Build history of the part. All positions in model axes, mm. A direction names the side the tool comes from. Give positions to 0.01 mm unless a question says otherwise; leave off trailing zeros. Loops run counter-clockwise (first coordinate to the right, second up) from the corner with the lowest first, then second, coordinate; pieces in that order, holes last.
1) Band-saw the part on A-A on x = -42. List the corners of the cut face in (y, z), then the cut area to 3 significant figures.
2) Wall check: line 1 (X direction, y = -0.5, z = 0.5); line 2 (X direction, y = -0.75, z = 0.75); line 3 (X direction, y = -1.75, z = 7.25). Give the ranges that are in metal, low to high.
3) 3-axis set-ups, long thin cutter, end or side, ignore diameter. For faces 3 (the cylindrical face through (-43.295, 0.318, 4.19)), 4 (the flat face through (-18, 2.236, 3)): which of +Z, -Z, +X, -X, +Y, -Y reach the whole face in a straight line?
4) Band-saw the part on C-C on z = -0.5. List the corners of the cut face in (x, y).
5) Band-saw the part on B-B on z = 6.25. List the corners of the cut face in (x, y), then the cut area to 3 significant figures.
6) Two-plate mould, pull along X, no slides. Class faces 1 (the flat face through (6, -4, -1.5)), 2 (the flat face through (-18, -5.764, 3)): +X half, -X half, draft (parallel to the pull), parting line (faces both ways), or undercut.
7) Flat gauge pins, fed straight in: P1, Ø1.5, axis at x = -29, z = 3, coming from the -Y side; P2, Ø3, axis at x = -37, z = 0, coming from the +Y side; P3, Ø5, axis at x = 5.5, z = 7, coming from the -Y side. Where does each tip first touch, or does it go through?
8) Band-saw the part on D-D on y = -4.5. List the corners of the cut face in (x, z), then the cut area to 3 significant figures.
```python
from build123d import *

# Parameters (mm, degrees)
SKETCH2_R           = 2.1
BOSS_EXTRUDE1_DEPTH = 7
SKETCH3_R           = 5
SKETCH3_R_2         = 2.1
BOSS_EXTRUDE2_DEPTH = 1.5
SKETCH4_R           = 5
SKETCH4_R_2         = 2.1
BOSS_EXTRUDE3_DEPTH = 1.5


with BuildPart() as part:
    # Sketch2 → Boss-Extrude1 (new body)
    with BuildSketch(Plane.XY):
        with BuildLine():
            ThreePointArc((-40.021658011, 2.236067977), (-48.021658011, -1.763932023), (-40.021658011, -5.763932023))
            Line((-40.021658011, -5.763932023), (-40.021658011, 2.236067977))
        make_face()
        with Locations((-43.021658011, -1.763932023)):
            Circle(SKETCH2_R, mode=Mode.SUBTRACT)
        with BuildLine():
            Line((-40.021658011, 2.236067977), (-40.021658011, -5.763932023))
            ThreePointArc((-40.021658011, -5.763932023), (-38.549522056, -4), (-38.021658011, -1.763932023))
            ThreePointArc((-38.021658011, -1.763932023), (-38.549522056, 0.472135955), (-40.021658011, 2.236067977))
        make_face()
        with BuildLine():
            ThreePointArc((-38.021658011, -1.763932023), (-38.549522056, -4), (-40.021658011, -5.763932023))
            Line((-40.021658011, -5.763932023), (3.978341989, -5.763932023))
            ThreePointArc((3.978341989, -5.763932023), (1.978341989, -1.763932023), (3.978341989, 2.236067977))
            Line((3.978341989, 2.236067977), (-40.021658011, 2.236067977))
            ThreePointArc((-40.021658011, 2.236067977), (-38.549522056, 0.472135955), (-38.021658011, -1.763932023))
        make_face()
        with BuildLine():
            Line((3.978341989, 2.236067977), (3.978341989, -5.763932023))
            ThreePointArc((3.978341989, -5.763932023), (9.214409967, -6.236067977), (11.978341989, -1.763932023))
            ThreePointArc((11.978341989, -1.763932023), (9.214409967, 2.708203932), (3.978341989, 2.236067977))
        make_face()
        with Locations((6.978341989, -1.763932023)):
            Circle(SKETCH2_R, mode=Mode.SUBTRACT)
        with BuildLine():
            ThreePointArc((3.978341989, 2.236067977), (1.978341989, -1.763932023), (3.978341989, -5.763932023))
            Line((3.978341989, -5.763932023), (3.978341989, 2.236067977))
        make_face()
    extrude(amount=BOSS_EXTRUDE1_DEPTH)

    # Sketch3 → Boss-Extrude2 (add)
    with BuildSketch(Plane.XY.offset(7)):
        with Locations((-43.021658011, -1.763932023)):
            Circle(SKETCH3_R)
        with Locations((-43.021658011, -1.763932023)):
            Circle(SKETCH3_R_2, mode=Mode.SUBTRACT)
    extrude(amount=BOSS_EXTRUDE2_DEPTH)

    # Sketch4 → Boss-Extrude3 (add)
    with BuildSketch(Plane(origin=(0, 0, 0), x_dir=(-1, 0, 0), z_dir=(0, 0, -1))):
        with Locations((-6.978341989, -1.763932023)):
            Circle(SKETCH4_R)
        with Locations((-6.978341989, -1.763932023)):
            Circle(SKETCH4_R_2, mode=Mode.SUBTRACT)
    extrude(amount=BOSS_EXTRUDE3_DEPTH)


solid = part.part
```
Findings below:
1. outline: (-6.66, 0) - (-3.6, 0) - (-3.6, 8.5) - (-6.66, 8.5) - close; (0.07, 0) - (3.13, 0) - (3.13, 8.5) - (0.07, 8.5) - close
1. area: 52.0 mm2
2. line 1: x = -47.86 to -44.7, -41.34 to 5.3, 8.66 to 11.82
2. line 2: x = -47.92 to -44.86, -41.18 to 5.14, 8.82 to 11.87
2. line 3: x = -48.02 to -45.12, -40.92 to -38.02
3. face 3: +Z, -Z
3. face 4: +Z, -Z, +Y
4. outline: circle Ø10 at (6.98, -1.76); hole circle Ø4.2 at (6.98, -1.76)
5. outline: (-40.02, -5.76) - (3.98, -5.76) arc R5 ccw (long way) to (3.98, 2.24) - (-40.02, 2.24) arc R5 ccw (long way) to start; hole circle Ø4.2 at (-43.02, -1.76); hole circle Ø4.2 at (6.98, -1.76)
5. area: 459 mm2
6. face 1: draft
6. face 2: undercut
7. P1: stops at y = -5.76
7. P2: stops at y = 2.24
7. P3: stops at y = -6.76
8. outline: (-47.21, 0) - (2.79, 0) - (2.79, -1.5) - (11.16, -1.5) - (11.16, 7) - (-38.84, 7) - (-38.84, 8.5) - (-47.21, 8.5) - close
8. area: 434 mm2
